Geometry: final body of the model. Coordinates: model frame, mm. Give positions to 0.01 mm unless a question says otherwise; leave off trailing zeros. Loops run counter-clockwise (first coordinate to the right, second up) from the corner with the lowest first, then second, coordinate; pieces in that order, holes last. Notation, with made-up numbers: (-24, 45.25) - (-20, 45.25) arc R19 cw to (-20, 75.25) - close; hole circle Ø7 at (28, 71). An arc over 180 degrees is marked (long way). Use one line per item in the form item = value.
```python
from build123d import *

# Parameters (mm, degrees)
F1_DEPTH = 0.5


with BuildPart() as f1:
    # F0 (on Front) → F1 (new body)
    with BuildSketch(Plane.XZ):
        with BuildLine():
            ThreePointArc((73.980978, 0), (74.14326, -0.003314), (74.305542, 0))
            Line((74.305542, 0), (73.980978, 0))
        make_face()
        with BuildLine():
            Line((73.980978, 0), (74.305542, 0))
            ThreePointArc((74.305542, 0), (77.011037, 1.219003), (78.118579, 3.972005))
            ThreePointArc((78.118579, 3.972005), (77.011037, 6.725007), (74.305542, 7.944011))
            ThreePointArc((74.305542, 7.944011), (70.171255, 4.134287), (73.980978, 0))
        make_face()
        with BuildLine():
            Line((-70.694458, 0), (73.980978, 0))
            ThreePointArc((73.980978, 0), (70.171255, 4.134287), (74.305542, 7.944011))
            Line((74.305542, 7.944011), (48.821039, 23.772469))
            Line((48.821039, 23.772469), (-70.694458, 13))
            Line((-70.694458, 13), (-70.694458, 0))
        make_face()
    extrude(amount=F1_DEPTH)


solid = f1.part
```
(1) Cut plane B-B (x = 36). Return the cut outline in (y, z).
Solution:
outline = (-0.5, 0) - (0, 0) - (0, 22.62) - (-0.5, 22.62) - close
(2) Pin query (flat end, axial travel): P1, Ø1, axis at x = 40, z = 14.5, coming from the +Y side. Return the tip coordinate at first contact, or that it passes through.
Solution:
P1 = 0
(3) Cut plane A-A (y = -0.4). Return the cut outline in (x, z), plus the area to 3 significant figures.
Solution:
outline = (-70.69, 0) - (73.98, 0) arc R3.98 ccw to (74.31, 0) arc R3.98 ccw to (78.12, 3.97) arc R3.98 ccw to (74.31, 7.94) - (48.82, 23.77) - (-70.69, 13) - close
area = 2,630 mm2
(4) Material intervals for L1, parallel to Z at x = 31, y = -0.45; L2, parallel to Z at x = 8.5, y = -0.15; L3, parallel to X at y = -0.1, z = 2.5, sorted ascending. Write a range as from..to.
Solution:
L1 = 0..22.17
L2 = 0..20.14
L3 = -70.69..77.84
(5) Cut plane C-C (z = 9.5). Return the cut outline in (x, y).
Solution:
outline = (-70.69, -0.5) - (71.8, -0.5) - (71.8, 0) - (-70.69, 0) - close
